```python
from build123d import *

# Parameters (mm, degrees)
BOSS_EXTRUDE1_DEPTH = 5
BOSS_EXTRUDE2_DEPTH = 3
SKETCH3_W           = 160
SKETCH3_H           = 12
BOSS_EXTRUDE3_DEPTH = 35
FILLET5_R           = 3
CUT_EXTRUDE1_DEPTH  = 241.425192154
FILLET12_R          = 5
FILLET13_R          = 2
FILLET14_R          = 2
FILLET15_R          = 2


# Some blends are built 0.0001 mm under size
with BuildPart() as part:
    # Sketch1 → Boss-Extrude1 (new body)
    with BuildSketch(Plane(origin=(0, 0, 0), x_dir=(1, 0, 0), z_dir=(0, 1, 0))):
        with BuildLine():
            Line((-80, -162), (80, -162))
            Line((80, -162), (80, -150))
            Line((80, -150), (3, -150))
            Line((3, -150), (3, -19.773719933))
            ThreePointArc((3, -19.773719933), (10.684156309, -16.90706373), (16.571665535, -11.197316705))
            Line((16.571665535, -11.197316705), (37.844608185, -22.65513623))
            ThreePointArc((37.844608185, -22.65513623), (73.921408989, -39.814809694), (39.741412764, -19.133470092))
            Line((39.741412764, -19.133470092), (18.468470115, -7.675650567))
            ThreePointArc((18.468470115, -7.675650567), (17.170912293, 10.25474383), (2, 19.899748742))
            Line((2, 19.899748742), (2, 32.406243273))
            ThreePointArc((2, 32.406243273), (0, 72.305992015), (-2, 32.406243273))
            Line((-2, 32.406243273), (-2, 19.899748742))
            ThreePointArc((-2, 19.899748742), (-15.477380683, 12.666913088), (-19.902285109, -1.97460058))
            Line((-19.902285109, -1.97460058), (-43.255678368, -6.68568275))
            ThreePointArc((-43.255678368, -6.68568275), (-81.972040815, -16.536227331), (-42.464692112, -10.606695469))
            Line((-42.464692112, -10.606695469), (-19.111298852, -5.895613299))
            ThreePointArc((-19.111298852, -5.895613299), (-13.052886469, -15.153288581), (-3, -19.773719933))
            Line((-3, -19.773719933), (-3, -150))
            Line((-3, -150), (-80, -150))
            Line((-80, -150), (-80, -162))
        make_face()
    extrude(amount=BOSS_EXTRUDE1_DEPTH)

    # Sketch2 → Boss-Extrude2 (add, symmetric)
    with BuildSketch(Plane(origin=(0, 0, 0), x_dir=(0, 0, -1), z_dir=(1, 0, 0))):
        Polygon((-150, 5), (-150, 40), (-114.292857857, 5), align=None)
    extrude(amount=BOSS_EXTRUDE2_DEPTH, both=True)

    # Sketch3 → Boss-Extrude3 (add)
    with BuildSketch(Plane(origin=(0, 5, 0), x_dir=(1, 0, 0), z_dir=(0, 1, 0))):
        with Locations((0, -156)):
            Rectangle(SKETCH3_W, SKETCH3_H)
    extrude(amount=BOSS_EXTRUDE3_DEPTH)

    # Fillet5
    fillet5_edges = [part.edges().sort_by_distance(p)[0] for p in [
        (0, 5, 114.292857857),
    ]]
    fillet(fillet5_edges, radius=FILLET5_R)

    # Sketch4 → Cut-Extrude1 (cut, through all)
    with BuildSketch(Plane(origin=(0, 0, 150), x_dir=(-1, 0, 0), z_dir=(0, 0, -1))):
        Polygon((80, 0), (3, 40), (80, 40), align=None)
        Polygon((-80, 40), (-80, 0), (-3, 40), align=None)
    extrude(amount=-CUT_EXTRUDE1_DEPTH, mode=Mode.SUBTRACT)

    # Fillet12
    # the kernel refuses this fillet: 5 mm, written as the material it adds along each edge
    with BuildSketch(Plane(origin=(-3, 0, 150), x_dir=(0, 0, -1), z_dir=(0, 1, 0))) as fillet12_piece_1_section:
        with BuildLine():
            CenterArc((FILLET12_R, FILLET12_R), FILLET12_R, 180, 90)
            Line((0, FILLET12_R), (0, 0))
            Line((0, 0), (FILLET12_R, 0))
        make_face()
    fillet12_piece_1 = extrude(amount=52.5, mode=Mode.PRIVATE)
    fillet12_piece_1 = split(fillet12_piece_1, bisect_by=Plane(origin=(-4.134914786, 29.296214811, 139.07995488), z_dir=(0, -0.7141428428542851, 0.7)), keep=Keep.TOP, mode=Mode.PRIVATE)
    fillet12_piece_1 = split(fillet12_piece_1, bisect_by=Plane(origin=(-12.366288086, 35.1343958, 148.888985243), z_dir=(0.4609898282276015, -0.8874054193381323, 0)), keep=Keep.TOP, mode=Mode.PRIVATE)
    add(fillet12_piece_1)
    with BuildSketch(Plane(origin=(3, 0, 150), x_dir=(0, 0, -1), z_dir=(0, 1, 0))) as fillet12_piece_2_section:
        with BuildLine():
            CenterArc((FILLET12_R, -FILLET12_R), FILLET12_R, 90, 90)
            Line((0, -FILLET12_R), (0, 0))
            Line((0, 0), (FILLET12_R, 0))
        make_face()
    fillet12_piece_2 = extrude(amount=52.5, mode=Mode.PRIVATE)
    fillet12_piece_2 = split(fillet12_piece_2, bisect_by=Plane(origin=(4.134914786, 29.296214811, 139.07995488), z_dir=(0, -0.7141428428542851, 0.7)), keep=Keep.TOP, mode=Mode.PRIVATE)
    fillet12_piece_2 = split(fillet12_piece_2, bisect_by=Plane(origin=(12.366288086, 35.1343958, 148.888985243), z_dir=(-0.4609898282276015, -0.8874054193381323, 0)), keep=Keep.TOP, mode=Mode.PRIVATE)
    add(fillet12_piece_2)

    # Fillet13
    fillet13_edges = [part.edges().sort_by_distance(p)[0] for p in [
        (-30.787995482, 0, 8.251154384),
        (-31.578981738, 0, 4.330141665),
        (-31.578981738, 5, 4.330141665),
        (-30.787995482, 5, 8.251154384),
    ]]
    fillet(fillet13_edges, radius=FILLET13_R - 0.0001)  # a hair under: the kernel refuses the full size

    # Fillet14
    fillet14_edges = [part.edges().sort_by_distance(p)[0] for p in [
        (27.20813686, 5, 16.926226468),
        (29.104941439, 5, 13.40456033),
        (29.104941439, 0, 13.40456033),
        (27.20813686, 0, 16.926226468),
    ]]
    fillet(fillet14_edges, radius=FILLET14_R - 0.0001)  # a hair under: the kernel refuses the full size

    # Fillet15
    fillet15_edges = [part.edges().sort_by_distance(p)[0] for p in [
        (-2, 0, -26.152996008),
        (2, 0, -26.152996008),
        (2, 5, -26.152996008),
        (-2, 5, -26.152996008),
    ]]
    fillet(fillet15_edges, radius=FILLET15_R - 0.0001)  # a hair under: the kernel refuses the full size


solid = part.part
```
Design review of the part built by this model. Coordinates are the model's own, in mm. A direction names the side the tool comes from. Give positions to 0.01 mm unless a question says otherwise; leave off trailing zeros. Write each loop counter-clockwise with the first axis right and the second up, starting at its lowest first coordinate (ties: lowest second). Pieces come first, ordered by that corner, then holes. Notation, with made-up numbers: (5.25, -4.5) - (61.25, -4.5) arc R19 cw to (61.25, 9.5) - close; hole circle Ø4 at (31, -18.5). An arc over 180 degrees is marked (long way). Return JSON: item names as keys, results as strings. Group by question number.
(1) We need section A-A, the plane x = -69.5. Give the boundary of the cut face in (y, z).
(2) We need section B-B, the plane x = -13. Give the boundary of the cut face in (y, z).
(3) We need section C-C, the plane y = 22.5. Give the boundary of the cut face in (x, z).
(4) Insertion check: pin 1 (12 mm diameter, centred on y = 14.5, z = -10, fed in from +X); pin 2 (17.5 mm diameter, centred on y = 10.5, z = 92.5, fed in from +X); pin 3 (0.8 mm diameter, centred on y = 2.5, z = -28, fed in from +X); pin 4 (6 mm diameter, centred on x = 18.5, y = 9, fed in from -Z). Each pin has a flat end and moves straight along its axis. Give the tip position at first contact, or say it passes through.
(5) Machinability: for faces 5 (the cylindrical face through (-30.74, 4.43, 7.63)), 6 (the flat face through (-2, 0, 36)), 7 (the cylindrical face through (-30.74, 0.57, 7.63)), 8 (the flat face through (-30.951, 2.493, 8.284)), which of the approach directions +Z, -Z, +X, -X, +Y, -Y give a long, thin tool a straight path to every point of the face, cutting with its end or side? Answer none if there is none.
(6) Mouldability with a two-part tool opening along Z and no side actions: class faces 1 (the flat face through (-31.42, 2.49, 4.3)), 2 (the flat face through (-1, 15, 162)), 3 (the cylindrical face through (-15.319, 2.465, -12.858)), 4 (the flat face through (-29, 10, 150)) as +Z half, -Z half, draft (parallel to the pull), parting line (faces both ways), or undercut.
(7) To check wall thickness, follow probe 1 along X at (y, z) = (2.5, 14.5); probe 2 along Z at (x, y) = (45, 17); probe 3 along X at (y, z) = (10, 121). State the ranges of each line that lie inside material, in increasing order.
(8) We need section D-D, the plane x = 53.5. Give the boundary of the cut face in (y, z).
Reported:
{
 "1": {"outline": "(0, -6.1) - (5, -6.1) - (5, 31.27) - (0, 31.27) - close; (0, 150) - (5.45, 150) - (5.45, 162) - (0, 162) - close"},
 "2": {"outline": "(0, -67.5) - (5, -67.5) - (5, -37.11) - (0, -37.11) - close; (0, -15.2) - (5, -15.2) - (5, 15.2) - (0, 15.2) - close; (0, 150) - (34.81, 150) - (34.81, 162) - (0, 162) - close"},
 "3": {"outline": "(-36.69, 150) - (-8, 150) arc R5 cw to (-3, 145) - (-3, 132.15) - (3, 132.15) - (3, 145) arc R5 cw to (8, 150) - (36.69, 150) - (36.69, 162) - (-36.69, 162) - close"},
 "4": {"pin 1": "passes through", "pin 2": "stops at x = 3", "pin 3": "stops at x = 2", "pin 4": "stops at z = 150"},
 "5": {"face 5": "+Y", "face 6": "+Z, -Z, +X, -X, -Y", "face 7": "-Y", "face 8": "+Y, -Y"},
 "6": {"face 1": "-Z half", "face 2": "+Z half", "face 3": "undercut", "face 4": "undercut"},
 "7": {"probe 1": "x = -82.27 to -42.46, -13.77 to 13.77, 22.7 to 31.14, 44.09 to 68.54", "probe 2": "z = 150 to 162", "probe 3": "x = -3 to 3"},
 "8": {"outline": "(0, 10.53) - (5, 10.53) - (5, 50.13) - (0, 50.13) - close; (0, 150) - (13.77, 150) - (13.77, 162) - (0, 162) - close"}
}
